Read the model definition and answer for the solid it produces. Units are mm, in the model's axes. A direction names the side the tool comes from. Give positions to 0.01 mm unless a question says otherwise; leave off trailing zeros. Write each loop counter-clockwise with the first axis right and the second up, starting at its lowest first coordinate (ties: lowest second). Pieces come first, ordered by that corner, then holes. Notation, with made-up numbers: M -21,89.25 L 23,89.25 A11 ccw 23,94.25 Z; hole C 38,-21 d8. An arc over 180 degrees is marked long. Use a Markdown table: item, result. Add a question column.
Item 1: For faces 4 (the flat face through (5.5, 10.3, 2.3)), 5 (the flat face through (7.367, 6.579, 2.337)), determine the directions among +Z, -Z, +X, -X, +Y, -Y from which every point of the face is accessible in a straight line to the end or side of a thin tool.
Item 2: A cutting plane is placed at C-C on y = -4. Determine the outline of the cut face in (x, z).
Item 3: Consider probe 1 along Y at (x, z) = (0, 1.7) (3 decimals); probe 2 along Y at (x, z) = (3.75, 1.1); probe 3 along X at (y, z) = (6, 1.85). Determine where each line is inside the solid, lowest interval first. Write a range as [from, to].
Item 4: A cutting plane is placed at D-D on x = 8. Determine the outline of the cut face in (y, z).
Item 5: A cutting plane is placed at A-A on z = 4.05. Determine the outline of the cut face in (x, y) (3 decimals), then the cut area to 3 significant figures.
Item 6: Given P1, Ø1, axis at x = 1.5, z = 2.5, coming from the -Y side; P2, Ø1.5, axis at x = 7, z = 2.5, coming from the +Y side, each flat-ended and moving along its own axis, determine where each tip first touches the part or whether it passes through.
Item 7: A cutting plane is placed at B-B on x = 0. Determine the outline of the cut face in (y, z) (3 decimals).
Item 8: The mould has two halves that part along X. Classify faces 1 (the flat face through (-4, 7, 0)), 2 (the flat face through (-7.373, 6.609, 2.337)), 3 (the cylindrical face through (-6.01, -4.61, 2.34)): pulls with the +X half, pulls with the -X half, needs draft (parallel to the pull), parting line crosses it, or undercut.
from build123d import *

# Parameters (mm, degrees)
F0_R     = 7.575
F1_DEPTH = 4.74


with BuildPart() as f1:
    # F0 (on Top) → F1 (new body)
    with BuildSketch(Plane.XY):
        with BuildLine():
            ThreePointArc((-7.128206, 5.534247), (-2.925035, -8.537176), (9.024367, 0))
            ThreePointArc((9.024367, 0), (8.537176, 2.925035), (7.128205, 5.534247))
            ThreePointArc((7.128205, 5.534247), (0, 9.024367), (-7.128206, 5.534247))
        make_face()
        Circle(F0_R, mode=Mode.SUBTRACT)
        with BuildLine():
            ThreePointArc((-7.128206, 5.534247), (0, 9.024367), (7.128205, 5.534247))
            Line((7.128205, 5.534247), (7.611939, 7.653624))
            Line((7.611939, 7.653624), (3.387632, 12.950739))
            Line((3.387632, 12.950739), (-3.387632, 12.950739))
            Line((-3.387632, 12.950739), (-7.61194, 7.653624))
            Line((-7.61194, 7.653624), (-7.128206, 5.534247))
        make_face()
    extrude(amount=F1_DEPTH)


solid = f1.part
Filled in:
| question | item | result |
|---|---|---|
| 1 | face 4 | +Z, -Z, +X, +Y |
| 1 | face 5 | +Z, -Z, +X |
| 2 | outline | M -8.09,0 L -6.43,0 L -6.43,4.74 L -8.09,4.74 Z; M 6.43,0 L 8.09,0 L 8.09,4.74 L 6.43,4.74 Z |
| 3 | probe 1 | [-9.024, -7.575], [7.575, 12.951] |
| 3 | probe 2 | [-8.21, -6.58], [6.58, 12.5] |
| 3 | probe 3 | [-7.23, -4.62], [4.62, 7.23] |
| 4 | outline | M -4.18,0 L 4.18,0 L 4.18,4.74 L -4.18,4.74 Z |
| 5 | outline | M -7.612,7.654 L -7.128,5.534 A9.024 ccw long 9.024,0 A9.024 ccw 7.128,5.534 L 7.612,7.654 L 3.388,12.951 L -3.388,12.951 Z; hole C 0,0 d15.15 |
| 5 | area | 130 mm² |
| 6 | P1 | y = -8.97 |
| 6 | P2 | y = 9.36 |
| 7 | outline | M -9.024,0 L -7.575,0 L -7.575,4.74 L -9.024,4.74 Z; M 7.575,0 L 12.951,0 L 12.951,4.74 L 7.575,4.74 Z |
| 8 | face 1 | needs draft |
| 8 | face 2 | pulls with the -X half |
| 8 | face 3 | undercut |
